For this review, take the finished solid that the model builds, in its own axes (mm). Face numbers are marked on the shaded views. A direction names the side the tool comes from. Round coordinates to 2 decimals unless told otherwise and drop trailing zeros. Order: outer loops, then holes, each group sorted by start corner. A loop starts at its lowest first (then second) coordinate and runs counter-clockwise, first axis right, second up. Notation, with made-up numbers: (-3, 3.5) -> (22, 3.5) arc R9 ccw to (22, 18.5) -> close; hole circle Ø9 at (80, 31). An arc over 180 degrees is marked (long way). Use a Markdown table: item, result. Add a question column.
1) Consider section A-A (z = 0). State the section outline as (x, y) points.
2) Clearance check with flat-ended pins moving along their axes: P1, Ø8, axis at x = 6.5, y = 21.5, coming from the +Z side; P2, Ø1.2, axis at x = -8.75, z = 0, coming from the -Y side; P3, Ø8, axis at x = -9, y = 33, coming from the +Z side. State where each tip first meets the part, or that it passes through.
3) Draft analysis for pull direction Y (two halves, no side actions). For the marked faces 1, 2 and 3, state which applies: pulls with the +Y half, pulls with the -Y half, needs draft (parallel to the pull), parting line crosses it, or undercut.
4) Consider section B-B (z = 8.75). State the section outline as (x, y) points.
5) Consider section C-C (z = -8.5). Give the number of separate pieces and of enclosed holes in the cut face, plus the area to 3 significant figures.
6) Consider section D-D (y = 24). State the section outline as (x, z) points, plus the area to 3 significant figures.
7) Wall thickness on line 1 along Y through (x, z) = (0, -5.5); line 2 along X through (y, z) = (4.3, 0); line 3 along X through (y, z) = (17, 5): over which ranges is each line inside the solid? List them lowest first. Write a range as [from, to].
8) Machinability: for the marked faces 4 and 5, which of the approach directions +Z, -Z, +X, -X, +Y, -Y give a long, thin tool a straight path to every point of the face, cutting with its end or side? Answer none if there is none.
```python
from build123d import *

# Parameters (mm, degrees)
SKETCH1_W           = 33
SKETCH1_H           = 27
BOSS_EXTRUDE1_DEPTH = 46
SKETCH3_W           = 16.5
SKETCH3_H           = 41
CUT_EXTRUDE2_DEPTH  = 59.200085911
FILLET3_R           = 16.5
SKETCH9_W           = 13
SKETCH9_H           = 23
CUT_EXTRUDE4_DEPTH  = 9
SKETCH10_R          = 6.5
CUT_EXTRUDE5_DEPTH  = 56.12259065
SKETCH11_R          = 1
CUT_EXTRUDE6_DEPTH  = 8
BOSS_EXTRUDE7_DEPTH = 16.5
FILLET5_R           = 4
CUT_EXTRUDE7_DEPTH  = 4
SKETCH17_R          = 1.3
CUT_EXTRUDE8_DEPTH  = 1.75
SKETCH18_R          = 2.35
CUT_EXTRUDE9_DEPTH  = 1
SKETCH19_R          = 0.75
CUT_EXTRUDE10_DEPTH = 1.75


# Some blends are built 0.0001 mm under size
with BuildPart() as part:
    # Sketch1 → Boss-Extrude1 (new body)
    with BuildSketch(Plane(origin=(0, 0, 0), x_dir=(1, 0, 0), z_dir=(0, 1, 0))):
        Rectangle(SKETCH1_W, SKETCH1_H)
    extrude(amount=BOSS_EXTRUDE1_DEPTH)

    # Sketch3 → Cut-Extrude2 (cut, through all)
    with BuildSketch(Plane(origin=(16.5, 0, 0), x_dir=(0, 0, -1), z_dir=(1, 0, 0))):
        with Locations((-5.25, 25.5)):
            Rectangle(SKETCH3_W, SKETCH3_H)
    extrude(amount=-CUT_EXTRUDE2_DEPTH, mode=Mode.SUBTRACT)

    # Fillet3
    fillet3_edges = [part.edges().sort_by_distance(p)[0] for p in [
        (-16.5, 46, -8.25),
        (16.5, 46, -8.25),
    ]]
    fillet(fillet3_edges, radius=FILLET3_R - 0.0001)  # a hair under: the kernel refuses the full size

    # Sketch9 → Cut-Extrude4 (cut)
    with BuildSketch(Plane.XY.offset(-3)):
        with Locations((0, 23)):
            Rectangle(SKETCH9_W, SKETCH9_H)
    extrude(amount=-CUT_EXTRUDE4_DEPTH, mode=Mode.SUBTRACT)

    # Sketch10 → Cut-Extrude5 (cut, through all)
    with BuildSketch(Plane.XY.offset(-12)):
        with Locations((0, 28)):
            Circle(SKETCH10_R)
    extrude(amount=-CUT_EXTRUDE5_DEPTH, mode=Mode.SUBTRACT)

    # Sketch11 → Cut-Extrude6 (cut)
    with BuildSketch(Plane.XY.offset(-3)):
        with Locations((0, 36.8)):
            Circle(SKETCH11_R)
        with Locations((0, 9.2)):
            Circle(SKETCH11_R)
    extrude(amount=-CUT_EXTRUDE6_DEPTH, mode=Mode.SUBTRACT)

    # Sketch15 → Boss-Extrude7 (add)
    with BuildSketch(Plane.XY.offset(-3)):
        with BuildLine():
            Line((13.5, 5), (13.5, 29.5))
            ThreePointArc((13.5, 29.5), (9.545941546, 39.045941546), (0, 43))
            ThreePointArc((0, 43), (-9.545941546, 39.045941546), (-13.5, 29.5))
            Line((-13.5, 29.5), (-13.5, 5))
            Line((-13.5, 5), (-16.5, 5))
            Line((-16.5, 5), (-16.5, 29.5))
            ThreePointArc((-16.5, 29.5), (-11.66726189, 41.16726189), (0, 46))
            ThreePointArc((0, 46), (11.66726189, 41.16726189), (16.5, 29.5))
            Line((16.5, 29.5), (16.5, 5))
            Line((16.5, 5), (13.5, 5))
        make_face()
    extrude(amount=BOSS_EXTRUDE7_DEPTH)

    # Fillet5
    # the kernel refuses this fillet: 4 mm, written as the material it takes off along each edge
    with BuildSketch(Plane(origin=(16.5, 29.5, 13.5), x_dir=(0, 0, -1), z_dir=(0, -1, 0))) as fillet5_piece_1:
        with BuildLine():
            CenterArc((FILLET5_R, -FILLET5_R), FILLET5_R, 90, 90)
            Line((0, -FILLET5_R), (0, 0))
            Line((0, 0), (FILLET5_R, 0))
        make_face()
    extrude(amount=39.5, mode=Mode.SUBTRACT)
    with BuildSketch(Plane(origin=(-16.5, 29.5, 13.5), x_dir=(0, 0, -1), z_dir=(0, -1, 0))) as fillet5_piece_2:
        with BuildLine():
            CenterArc((FILLET5_R, FILLET5_R), FILLET5_R, 180, 90)
            Line((0, FILLET5_R), (0, 0))
            Line((0, 0), (FILLET5_R, 0))
        make_face()
    extrude(amount=39.5, mode=Mode.SUBTRACT)
    with BuildSketch(Plane(origin=(-16.5, -10, -13.5), x_dir=(0, 0, 1), z_dir=(0, 1, 0))) as fillet5_piece_3:
        with BuildLine():
            CenterArc((FILLET5_R, FILLET5_R), FILLET5_R, 180, 90)
            Line((0, FILLET5_R), (0, 0))
            Line((0, 0), (FILLET5_R, 0))
        make_face()
    extrude(amount=39.5001, mode=Mode.SUBTRACT)
    with BuildSketch(Plane(origin=(16.5, -10, -13.5), x_dir=(0, 0, 1), z_dir=(0, 1, 0))) as fillet5_piece_4:
        with BuildLine():
            CenterArc((FILLET5_R, -FILLET5_R), FILLET5_R, 90, 90)
            Line((0, -FILLET5_R), (0, 0))
            Line((0, 0), (FILLET5_R, 0))
        make_face()
    extrude(amount=39.5001, mode=Mode.SUBTRACT)
    with BuildSketch(Plane(origin=(0.0001, 29.5001, -13.5), x_dir=(1, 0, 0), z_dir=(0, -1, 0))) as fillet5_piece_5:
        with BuildLine():
            CenterArc((16.4999 - FILLET5_R, FILLET5_R), FILLET5_R, 270, 90)
            Line((16.4999 - FILLET5_R, 0), (16.4999, 0))
            Line((16.4999, 0), (16.4999, FILLET5_R))
        make_face()
    revolve(axis=Axis((0.0001, 29.5001, -13.5), (0, 0, 1)), revolution_arc=90, mode=Mode.SUBTRACT)
    with BuildSketch(Plane(origin=(0, 29.5, 13.5), x_dir=(-1, 0, 0), z_dir=(0, -1, 0))) as fillet5_piece_6:
        with BuildLine():
            CenterArc((16.5 - FILLET5_R, FILLET5_R), FILLET5_R, 270, 90)
            Line((16.5 - FILLET5_R, 0), (16.5, 0))
            Line((16.5, 0), (16.5, FILLET5_R))
        make_face()
    revolve(axis=Axis((0, 29.5, 13.5), (0, 0, -1)), revolution_arc=180, mode=Mode.SUBTRACT)
    with BuildSketch(Plane(origin=(0.0001, 46, -13.5), x_dir=(0, 0, 1), z_dir=(-1, 0, 0))) as fillet5_piece_7:
        with BuildLine():
            CenterArc((FILLET5_R, -FILLET5_R), FILLET5_R, 90, 90)
            Line((0, -FILLET5_R), (0, 0))
            Line((0, 0), (FILLET5_R, 0))
        make_face()
    extrude(amount=0.0002, mode=Mode.SUBTRACT)
    with BuildSketch(Plane(origin=(-0.0001, 29.5001, -13.5), x_dir=(-1, 0, 0), z_dir=(0, -1, 0))) as fillet5_piece_8:
        with BuildLine():
            CenterArc((16.4999 - FILLET5_R, -FILLET5_R), FILLET5_R, 0, 90)
            Line((16.4999 - FILLET5_R, 0), (16.4999, 0))
            Line((16.4999, 0), (16.4999, -FILLET5_R))
        make_face()
    revolve(axis=Axis((-0.0001, 29.5001, -13.5), (0, 0, -1)), revolution_arc=90, mode=Mode.SUBTRACT)

    # Sketch4 → Cut-Extrude7 (cut)
    with BuildSketch(Plane.XZ):
        with BuildLine():
            Line((0.133928571, 2.49641005), (14.09375, 1.747487035))
            ThreePointArc((14.09375, 1.747487035), (15.75, 0), (14.09375, -1.747487035))
            Line((14.09375, -1.747487035), (0.133928571, -2.49641005))
            ThreePointArc((0.133928571, -2.49641005), (0, -2.5), (-0.133928571, -2.49641005))
            Line((-0.133928571, -2.49641005), (-14.09375, -1.747487035))
            ThreePointArc((-14.09375, -1.747487035), (-15.75, 0), (-14.09375, 1.747487035))
            Line((-14.09375, 1.747487035), (-0.133928571, 2.49641005))
            ThreePointArc((-0.133928571, 2.49641005), (0, 2.5), (0.133928571, 2.49641005))
        make_face()
    extrude(amount=-CUT_EXTRUDE7_DEPTH, mode=Mode.SUBTRACT)

    # Sketch17 → Cut-Extrude8 (cut)
    with BuildSketch(Plane.XZ.offset(-4)):
        with Locations(Location((0, 0, 0), (0, 0, 270))):
            Circle(SKETCH17_R)
    extrude(amount=-CUT_EXTRUDE8_DEPTH, mode=Mode.SUBTRACT)

    # Sketch18 → Cut-Extrude9 (cut)
    with BuildSketch(Plane(origin=(0, 5, 0), x_dir=(1, 0, 0), z_dir=(0, 1, 0))):
        with Locations(Location((0, 0, 0), (0, 0, 270))):
            Circle(SKETCH18_R)
    extrude(amount=-CUT_EXTRUDE9_DEPTH, mode=Mode.SUBTRACT)

    # Sketch19 → Cut-Extrude10 (cut)
    with BuildSketch(Plane.XZ.offset(-4)):
        with Locations(Location((-8.75, 0, 0), (0, 0, 270))):
            Circle(SKETCH19_R)
        with Locations(Location((8.75, 0, 0), (0, 0, 270))):
            Circle(SKETCH19_R)
    extrude(amount=-CUT_EXTRUDE10_DEPTH, mode=Mode.SUBTRACT)


solid = part.part
```
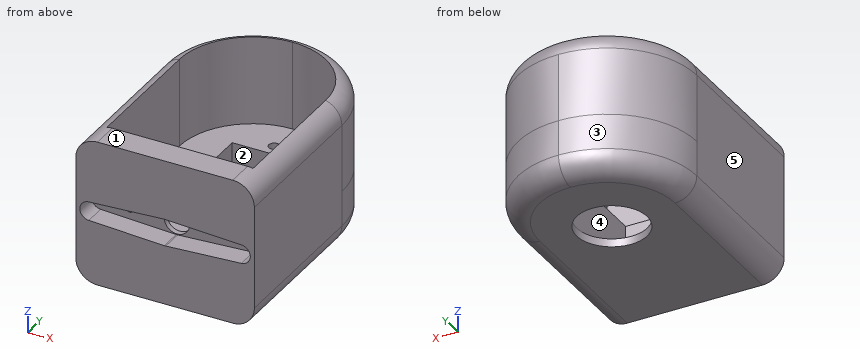
Results list:
| question | item | result |
|---|---|---|
| 1 | outline | (-16.5, 0) -> (-15.75, 0) -> (-15.75, 4) -> (-9.5, 4) -> (-9.5, 5) -> (-13.5, 5) -> (-13.5, 29.5) arc R13.5 cw to (13.5, 29.5) -> (13.5, 5) -> (9.5, 5) -> (9.5, 4) -> (15.75, 4) -> (15.75, 0) -> (16.5, 0) -> (16.5, 29.5) arc R16.5 ccw to (-16.5, 29.5) -> close; (-8, 4) -> (-2.35, 4) -> (-2.35, 5) -> (-8, 5) -> close; (2.35, 4) -> (8, 4) -> (8, 5) -> (2.35, 5) -> close |
| 2 | P1 | z = -3 |
| 2 | P2 | y = 39.24 |
| 2 | P3 | z = 13.37 |
| 3 | face 1 | needs draft |
| 3 | face 2 | undercut |
| 3 | face 3 | pulls with the +Y half |
| 4 | outline | (-16.5, 0) -> (16.5, 0) -> (16.5, 29.5) arc R16.5 ccw to (-16.5, 29.5) -> close; hole (-13.5, 5) -> (13.5, 5) -> (13.5, 29.5) arc R13.5 ccw to (-13.5, 29.5) -> close |
| 5 | separate pieces | 1 |
| 5 | enclosed holes | 3 |
| 5 | area | 1,100 mm2 |
| 6 | outline | (-16.5, -9.5) arc R4 ccw to (-12.5, -13.5) -> (-5.12, -13.5) -> (-5.12, -12) -> (-6.5, -12) -> (-6.5, -3) -> (-13.5, -3) -> (-13.5, 13.37) arc R4 ccw to (-16.5, 9.5) -> close; (5.12, -13.5) -> (12.5, -13.5) arc R4 ccw to (16.5, -9.5) -> (16.5, 9.5) arc R4 ccw to (13.5, 13.37) -> (13.5, -3) -> (6.5, -3) -> (6.5, -12) -> (5.12, -12) -> close |
| 6 | area | 299 mm2 |
| 7 | line 1 | [0, 8.2], [10.2, 11.5], [34.5, 35.8], [37.8, 46] |
| 7 | line 2 | [-16.5, -9.5], [-8, -2.35], [2.35, 8], [9.5, 16.5] |
| 7 | line 3 | [-16.5, -13.5], [13.5, 16.5] |
| 8 | face 4 | +Z |
| 8 | face 5 | +Z, -Z, -X, +Y, -Y |
